from build123d import *

# Parameters (mm, degrees)
SZKIC1_R                    = 5
DODANIE_WYCI_GNI_CIE1_DEPTH = 40
SZKIC3_R                    = 8
DODANIE_WYCI_GNI_CIE2_DEPTH = 5
SZKIC2_R                    = 8
DODANIE_WYCI_GNI_CIE3_DEPTH = 5


with BuildPart() as part:
    # Szkic1 → Dodanie-wyciągnięcie1 (new body)
    with BuildSketch(Plane(origin=(0, 0, 0), x_dir=(1, 0, 0), z_dir=(0, 1, 0))):
        Circle(SZKIC1_R)
    extrude(amount=DODANIE_WYCI_GNI_CIE1_DEPTH)

    # Szkic3 → Dodanie-wyciągnięcie2 (add)
    with BuildSketch(Plane.XZ):
        Circle(SZKIC3_R)
    extrude(amount=DODANIE_WYCI_GNI_CIE2_DEPTH)

    # Szkic2 → Dodanie-wyciągnięcie3 (add)
    with BuildSketch(Plane(origin=(0, 40, 0), x_dir=(1, 0, 0), z_dir=(0, 1, 0))):
        Circle(SZKIC2_R)
    extrude(amount=DODANIE_WYCI_GNI_CIE3_DEPTH)


solid = part.part
Input: part model. Units: mm. Frame: model coordinates. A direction names the side the tool comes from. Give positions to 0.01 mm unless a question says otherwise; leave off trailing zeros. Loops run counter-clockwise (first coordinate to the right, second up) from the corner with the lowest first, then second, coordinate; pieces in that order, holes last. Notation, with made-up numbers: (29, 21.25) - (69, 21.25) arc R25 ccw to (69, 49.25) - close; hole circle Ø2 at (56, 85.5). An arc over 180 degrees is marked (long way). Use CSV: the item, a comma, the result in double quotes. Start each with the question number.
Item 1: Section B-B on z = 0. Return loops of the section in (x, y), then the cut area to 3 significant figures.
Item 2: Contact query for flat-ended pins moving along their axis: P1, Ø1.5, axis at x = 2, y = 6, coming from the -Z side; P2, Ø2, axis at x = -2, y = 19, coming from the -Z side; P3, Ø3, axis at x = -6, y = 32.5, coming from the -Z side. Output: stop coordinate, or through.
Item 3: Line query: line 1 (Y direction, x = 3, z = -5.25); line 2 (Z direction, x = 0.25, y = 34); line 3 (X direction, y = 40.5, z = -3). Output: solid intervals per line, ascending.
Item 4: Section A-A on x = 7.25. Return loops of the section in (y, z), then the cut area to 3 significant figures.
Item 5: Mould query, pull axis Y, two halves, no side actions, for faces 3 (the cylindrical face through (-1.73, 42.46, 7.81)), 4 (the flat face through (5.2, 40, -0.1)), 5 (the flat face through (0, 45, 0)). Classes: pulls with the +Y half, pulls with the -Y half, needs draft (parallel to the pull), parting line crosses it, or undercut.
Item 6: Section C-C on x = 0. Return loops of the section in (y, z).
Item 7: Reachability of faces 1 (the flat face through (5.2, 0, 0.1)), 2 (the flat face through (0, -5, 0)) from +Z, -Z, +X, -X, +Y, -Y: full face, straight path, thin tool, end or side. Return the list, or none.
Item 8: Section D-D on y = 38. Return loops of the section in (x, z).
Ans:
1,outline,"(-8, -5) - (8, -5) - (8, 0) - (5, 0) - (5, 40) - (8, 40) - (8, 45) - (-8, 45) - (-8, 40) - (-5, 40) - (-5, 0) - (-8, 0) - close"
1,area,"560 mm2"
2,P1,"stops at z = -4.84"
2,P2,"stops at z = -4.9"
2,P3,"stops at z = -2.18"
3,line 1,"y = -5 to 0, 40 to 45"
3,line 2,"z = -4.99 to 4.99"
3,line 3,"x = -7.42 to 7.42"
4,outline,"(-5, -3.38) - (0, -3.38) - (0, 3.38) - (-5, 3.38) - close; (40, -3.38) - (45, -3.38) - (45, 3.38) - (40, 3.38) - close"
4,area,"67.6 mm2"
5,face 3,"needs draft"
5,face 4,"undercut"
5,face 5,"pulls with the +Y half"
6,outline,"(-5, -8) - (0, -8) - (0, -5) - (40, -5) - (40, -8) - (45, -8) - (45, 8) - (40, 8) - (40, 5) - (0, 5) - (0, 8) - (-5, 8) - close"
7,face 1,"none"
7,face 2,"+Z, -Z, +X, -X, -Y"
8,outline,"circle Ø10 at (0, 0)"
